from build123d import *

# Parameters (mm, degrees)
SKETCH2_W           = 100
SKETCH2_H           = 80
BOSS_EXTRUDE1_DEPTH = 10
SKETCH3_W           = 10
SKETCH3_H           = 10
BOSS_EXTRUDE2_DEPTH = 30
SKETCH4_W           = 5
SKETCH4_H           = 10
BOSS_EXTRUDE3_DEPTH = 10
SKETCH5_W           = 6
SKETCH5_H           = 6
BOSS_EXTRUDE4_DEPTH = 4
SKETCH6_R           = 1.5
CUT_EXTRUDE1_DEPTH  = 134.026313187
SKETCH7_W           = 100
SKETCH7_H           = 10
BOSS_EXTRUDE5_DEPTH = 45
SKETCH8_W           = 10
SKETCH8_H           = 10
BOSS_EXTRUDE6_DEPTH = 30
SKETCH9_W           = 5
SKETCH9_H           = 10
BOSS_EXTRUDE7_DEPTH = 10
SKETCH10_R          = 1.5
CUT_EXTRUDE2_DEPTH  = 166
SKETCH11_R          = 1.5
CUT_EXTRUDE3_DEPTH  = 10


with BuildPart() as part:
    # Sketch2 → Boss-Extrude1 (new body)
    with BuildSketch(Plane(origin=(0, 0, 0), x_dir=(1, 0, 0), z_dir=(0, 1, 0))):
        with Locations((50, 40)):
            Rectangle(SKETCH2_W, SKETCH2_H)
    extrude(amount=BOSS_EXTRUDE1_DEPTH)

    # Sketch3 → Boss-Extrude2 (add)
    with BuildSketch(Plane.XZ):
        with Locations((95, -5)):
            Rectangle(SKETCH3_W, SKETCH3_H)
        with Locations((5, -5)):
            Rectangle(SKETCH3_W, SKETCH3_H)
    extrude(amount=BOSS_EXTRUDE2_DEPTH)

    # Sketch4 → Boss-Extrude3 (add)
    with BuildSketch(Plane.XZ.offset(30)):
        with Locations((2.5, -5)):
            Rectangle(SKETCH4_W, SKETCH4_H)
        with Locations((97.5, -5)):
            Rectangle(SKETCH4_W, SKETCH4_H)
    extrude(amount=BOSS_EXTRUDE3_DEPTH)

    # Sketch5 → Boss-Extrude4 (add)
    with BuildSketch(Plane.XZ):
        with Locations((6, -13)):
            Rectangle(SKETCH5_W, SKETCH5_H)
        with Locations((95, -13)):
            Rectangle(SKETCH5_W, SKETCH5_H)
        with Locations((95, -77)):
            Rectangle(SKETCH5_W, SKETCH5_H)
        with Locations((6, -77)):
            Rectangle(SKETCH5_W, SKETCH5_H)
    extrude(amount=BOSS_EXTRUDE4_DEPTH)

    # Sketch6 → Cut-Extrude1 (cut, through all)
    with BuildSketch(Plane.XZ.offset(4)):
        with Locations(Location((6, -13, 0), (0, 0, 270))):
            Circle(SKETCH6_R)
        with Locations(Location((95, -13, 0), (0, 0, 270))):
            Circle(SKETCH6_R)
        with Locations(Location((95, -77, 0), (0, 0, 270))):
            Circle(SKETCH6_R)
        with Locations(Location((6, -77, 0), (0, 0, 270))):
            Circle(SKETCH6_R)
    extrude(amount=-CUT_EXTRUDE1_DEPTH, mode=Mode.SUBTRACT)

    # Sketch7 → Boss-Extrude5 (add)
    with BuildSketch(Plane(origin=(0, 0, -80), x_dir=(-1, 0, 0), z_dir=(0, 0, -1))):
        with Locations((-50, 5)):
            Rectangle(SKETCH7_W, SKETCH7_H)
    extrude(amount=BOSS_EXTRUDE5_DEPTH)

    # Sketch8 → Boss-Extrude6 (add)
    with BuildSketch(Plane.XZ):
        with Locations((5, -120)):
            Rectangle(SKETCH8_W, SKETCH8_H)
        with Locations((95, -120)):
            Rectangle(SKETCH8_W, SKETCH8_H)
    extrude(amount=BOSS_EXTRUDE6_DEPTH)

    # Sketch9 → Boss-Extrude7 (add)
    with BuildSketch(Plane.XZ.offset(30)):
        with Locations((2.5, -120)):
            Rectangle(SKETCH9_W, SKETCH9_H)
        with Locations((97.5, -120)):
            Rectangle(SKETCH9_W, SKETCH9_H)
    extrude(amount=BOSS_EXTRUDE7_DEPTH)

    # Sketch10 → Cut-Extrude2 (cut, through all)
    with BuildSketch(Plane.ZY):
        with Locations((-5, -35)):
            Circle(SKETCH10_R)
        with Locations((-120, -35)):
            Circle(SKETCH10_R)
    extrude(amount=-CUT_EXTRUDE2_DEPTH, mode=Mode.SUBTRACT)

    # Sketch11 → Cut-Extrude3 (cut)
    with BuildSketch(Plane.XZ):
        with Locations(Location((4, -106.5, 0), (0, 0, 270))):
            Circle(SKETCH11_R)
        with Locations(Location((4, -90, 0), (0, 0, 270))):
            Circle(SKETCH11_R)
        with Locations(Location((42.5, -106.5, 0), (0, 0, 270))):
            Circle(SKETCH11_R)
        with Locations(Location((42.5, -90, 0), (0, 0, 270))):
            Circle(SKETCH11_R)
    extrude(amount=-CUT_EXTRUDE3_DEPTH, mode=Mode.SUBTRACT)


solid = part.part
Input: part model. Units: mm. Frame: model coordinates. A direction names the side the tool comes from. Give positions to 0.01 mm unless a question says otherwise; leave off trailing zeros. Order: outer loops, then holes, each group sorted by start corner. A loop starts at its lowest first (then second) coordinate and runs counter-clockwise, first axis right, second up. Notation, with made-up numbers: (0, 54.5) -> (50, 54.5) arc R18 cw to (50, 61.5) -> close; hole circle Ø2 at (31, -38.5). An arc over 180 degrees is marked (long way). Use one line per item in the form item = value.
1) First-contact query: pin 1 Ø4 at (x, z) = (6, -13) entering from -Y; pin 2 Ø3.5 at (x, z) = (4, -90) entering from -Y; pin 3 Ø1.8 at (x, z) = (95, -77) entering from +Y. Flat tips, straight axial feed; report the tip coordinate or a pass-through.
Response values:
pin_1 = -4
pin_2 = 0
pin_3 = through
2) Section A-A, the plane z = -90. Return loops of the section in (x, y).
Response values:
outline = (0, 0) -> (2.5, 0) -> (2.5, 10) -> (0, 10) -> close; (5.5, 0) -> (41, 0) -> (41, 10) -> (5.5, 10) -> close; (44, 0) -> (100, 0) -> (100, 10) -> (44, 10) -> close
3) Section D-D, the plane x = 38. Return loops of the section in (y, z), and give its area (3 significant figures).
Response values:
outline = (0, -125) -> (10, -125) -> (10, 0) -> (0, 0) -> close
area = 1,250 mm^2
4) Mould query, pull axis Z, two halves, no side actions, for faces 1 (the flat face through (92, -2, -13)), 2 (the flat face through (7, -30, -5)). Classes: pulls with the +Z half, pulls with the -Z half, needs draft (parallel to the pull), parting line crosses it, or undercut.
Response values:
face_1 = undercut
face_2 = needs draft
5) Section C-C, the plane z = -13. Return loops of the section in (x, y), and give its area (3 significant figures).
Response values:
outline = (0, 0) -> (3, 0) -> (3, -4) -> (4.5, -4) -> (4.5, 10) -> (0, 10) -> close; (7.5, -4) -> (9, -4) -> (9, 0) -> (92, 0) -> (92, -4) -> (93.5, -4) -> (93.5, 10) -> (7.5, 10) -> close; (96.5, -4) -> (98, -4) -> (98, 0) -> (100, 0) -> (100, 10) -> (96.5, 10) -> close
area = 964 mm^2
6) Reachability of faces 3 (the flat face through (4.6, -4, -75.6)), 4 (the flat face through (51, 10, -62)), 5 (the flat face through (98, -2, -77)), 6 (the flat face through (10, -15, -5)) from +Z, -Z, +X, -X, +Y, -Y: full face, straight path, thin tool, end or side. Return the list, or none.
Response values:
face_3 = +X, -X, -Y
face_4 = +Z, -Z, +X, -X, +Y
face_5 = +X, -Y
face_6 = +Z, -Z, -Y
7) Line query: probe 1 along Z at (x, y) = (95, 1.25); probe 2 along X at (y, z) = (6.5, -13); probe 3 along X at (y, z) = (3.75, -106.5). Output: solid intervals per line, ascending.
Response values:
probe_1 = -125 to -78.5, -75.5 to -14.5, -11.5 to 0
probe_2 = 0 to 4.5, 7.5 to 93.5, 96.5 to 100
probe_3 = 0 to 2.5, 5.5 to 41, 44 to 100
8) Section B-B, the plane y = -18.5. Return loops of the section in (x, z).
Response values:
outline = (0, -125) -> (10, -125) -> (10, -115) -> (0, -115) -> close; (0, -10) -> (10, -10) -> (10, 0) -> (0, 0) -> close; (90, -125) -> (100, -125) -> (100, -115) -> (90, -115) -> close; (90, -10) -> (100, -10) -> (100, 0) -> (90, 0) -> close
